Geometry: final body of the model. Coordinates: model frame, mm. Face numbers are marked on the shaded views. A direction names the side the tool comes from. Coordinates: 2 decimals unless noted, no trailing zeros. Write each loop counter-clockwise with the first axis right and the second up, starting at its lowest first coordinate (ties: lowest second). Pieces come first, ordered by that corner, then holes. Notation, with made-up numbers: (3, 67) - (9, 67) arc R14 ccw to (9, 85) - close; hole circle Ø10 at (-33, -36). An arc over 180 degrees is marked (long way). Put each result on its own line as item: value.
```python
from build123d import *

# Parameters (mm, degrees)
SKETCH1_W           = 72
SKETCH1_H           = 47
BOSS_EXTRUDE1_DEPTH = 1.5
CUT_EXTRUDE1_DEPTH  = 1.5
SKETCH3_W           = 18
SKETCH3_H           = 10
BOSS_EXTRUDE2_DEPTH = 15
SKETCH4_W           = 51
SKETCH4_H           = 21
BOSS_EXTRUDE3_DEPTH = 4
SKETCH5_W           = 5.5
SKETCH5_H           = 8
BOSS_EXTRUDE4_DEPTH = 3
SKETCH6_R           = 3
BOSS_EXTRUDE5_DEPTH = 16
FILLET1_R           = 3


with BuildPart() as part:
    # Sketch1 → Boss-Extrude1 (new body)
    with BuildSketch(Plane(origin=(0, 0, 0), x_dir=(1, 0, 0), z_dir=(0, 1, 0))):
        with Locations((36, 23.5)):
            Rectangle(SKETCH1_W, SKETCH1_H)
    extrude(amount=BOSS_EXTRUDE1_DEPTH)

    # Sketch2 → Cut-Extrude1 (cut)
    with BuildSketch(Plane(origin=(0, 1.5, 0), x_dir=(1, 0, 0), z_dir=(0, 1, 0))):
        with BuildLine():
            ThreePointArc((67, 44), (67.585786438, 42.585786438), (69, 42))
            Line((69, 42), (69, 44))
            Line((69, 44), (67, 44))
        make_face()
        with BuildLine():
            Line((69, 44), (69, 42))
            ThreePointArc((69, 42), (70.414213562, 42.585786438), (71, 44))
            ThreePointArc((71, 44), (69, 46), (67, 44))
            Line((67, 44), (69, 44))
        make_face()
        with BuildLine():
            ThreePointArc((69, 5), (67.585786438, 4.414213562), (67, 3))
            Line((67, 3), (69, 3))
            Line((69, 3), (69, 5))
        make_face()
        with BuildLine():
            Line((69, 3), (67, 3))
            ThreePointArc((67, 3), (69, 1), (71, 3))
            ThreePointArc((71, 3), (70.414213562, 4.414213562), (69, 5))
            Line((69, 5), (69, 3))
        make_face()
        with BuildLine():
            Line((3, 5), (3, 3))
            Line((3, 3), (5, 3))
            ThreePointArc((5, 3), (4.414213562, 4.414213562), (3, 5))
        make_face()
        with BuildLine():
            Line((5, 3), (3, 3))
            Line((3, 3), (3, 5))
            ThreePointArc((3, 5), (1.585786438, 1.585786438), (5, 3))
        make_face()
        with BuildLine():
            ThreePointArc((5, 44), (1.585786438, 45.414213562), (3, 42))
            Line((3, 42), (3, 44))
            Line((3, 44), (5, 44))
        make_face()
        with BuildLine():
            Line((3, 44), (3, 42))
            ThreePointArc((3, 42), (4.414213562, 42.585786438), (5, 44))
            Line((5, 44), (3, 44))
        make_face()
    extrude(amount=-CUT_EXTRUDE1_DEPTH, mode=Mode.SUBTRACT)

    # Sketch3 → Boss-Extrude2 (add)
    with BuildSketch(Plane(origin=(0, 1.5, 0), x_dir=(1, 0, 0), z_dir=(0, 1, 0))):
        with Locations((19, 7)):
            Rectangle(SKETCH3_W, SKETCH3_H)
    extrude(amount=BOSS_EXTRUDE2_DEPTH)

    # Sketch4 → Boss-Extrude3 (add)
    with BuildSketch(Plane(origin=(0, 1.5, 0), x_dir=(1, 0, 0), z_dir=(0, 1, 0))):
        with Locations((29.5, 29.5)):
            Rectangle(SKETCH4_W, SKETCH4_H)
    extrude(amount=BOSS_EXTRUDE3_DEPTH)

    # Sketch5 → Boss-Extrude4 (add)
    with BuildSketch(Plane(origin=(0, 5.5, 0), x_dir=(1, 0, 0), z_dir=(0, 1, 0))):
        with Locations((5.25, 28.406225208)):
            Rectangle(SKETCH5_W, SKETCH5_H)
    extrude(amount=BOSS_EXTRUDE4_DEPTH)

    # Sketch6 → Boss-Extrude5 (add)
    with BuildSketch(Plane.XZ):
        with Locations(Location((58, -39, 0), (0, 0, 270))):
            Circle(SKETCH6_R)
    extrude(amount=BOSS_EXTRUDE5_DEPTH)

    # Fillet1
    fillet1_edges = [part.edges().sort_by_distance(p)[0] for p in [
        (58, -16, -36),
    ]]
    fillet(fillet1_edges, radius=FILLET1_R)


solid = part.part
```
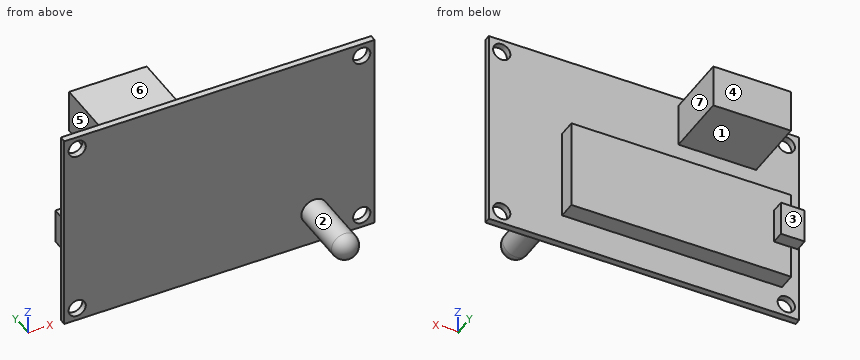
1. Section query D-D (x = 58). Return loops of the section in (y, z).
Answer below:
outline: (-13, -42) - (0, -42) - (0, -47) - (1.5, -47) - (1.5, 0) - (0, 0) - (0, -36) - (-13, -36) arc R3 ccw to start
2. Mould query, pull axis Z, two halves, no side actions, for the marked faces 1, 2 and 3. Classes: +Z half, -Z half, draft (parallel to the pull), parting line (faces both ways), or undercut.
Answer below:
face 1: undercut
face 2: parting line
face 3: draft
3. Section query B-B (z = -39). Return loops of the section in (x, y), then the cut area to 3 significant figures.
Answer below:
outline: (0, 0) - (55, 0) - (55, -13) arc R3 ccw to (61, -13) - (61, 0) - (72, 0) - (72, 1.5) - (55, 1.5) - (55, 5.5) - (4, 5.5) - (4, 1.5) - (0, 1.5) - close
area: 404 mm²
4. Section query C-C (y = -12). Return loops of the section in (x, z).
Answer below:
outline: circle Ø6 at (58, -39)
5. Ray query, probe 1 along Z at (x, y) = (3, 0.9); probe 2 along X at (y, z) = (0.65, -44); probe 3 along X at (y, z) = (4, -21). Return the intervals inside material, ascending. Write a range as from..to.
Answer below:
probe 1: z = -47..-46, -42..-5, -1..0
probe 2: x = 0..1, 5..67, 71..72
probe 3: x = 4..55
6. Pin query (flat end, axial travel): pin 1 Ø8 at (x, z) = (11, -11.5) entering from -Y; pin 2 Ø6 at (x, z) = (4, -29.5) entering from +Y; pin 3 Ø6 at (y, z) = (3.5, -18.5) entering from +X; pin 4 Ø3 at (y, z) = (11, -6) entering from +X. Return the tip coordinate at first contact, or that it passes through.
Answer below:
pin 1: stops at y = 0
pin 2: stops at y = 8.5
pin 3: stops at x = 72
pin 4: stops at x = 28
7. Set-up query: the marked faces 4, 5, 6 and 7. Return all of +Z, -Z, +X, -X, +Y, -Y with unobstructed straight access to the full face (end or side cutting, diameter ignored); none if empty.
Answer below:
face 4: +Z, -Z, +X, -X, +Y
face 5: +Z, -X, +Y
face 6: +Z, +X, -X, +Y
face 7: +Z, +X, +Y
8. Section query A-A (x = 29.5). Return loops of the section in (y, z), then the cut area to 4 significant figures.
Answer below:
outline: (0, -47) - (1.5, -47) - (1.5, -40) - (5.5, -40) - (5.5, -19) - (1.5, -19) - (1.5, 0) - (0, 0) - close
area: 154.5 mm²
